Read the model definition and answer for the solid it produces. Units are mm, in the model's axes. A direction names the side the tool comes from. Coordinates: 2 decimals unless noted, no trailing zeros. Write each loop counter-clockwise with the first axis right and the second up, starting at its lowest first coordinate (ties: lowest second). Pieces come first, ordered by that corner, then holes. Notation, with made-up numbers: (71, 19.5) - (130, 19.5) arc R18 cw to (130, 41.5) - close; hole circle Ø1 at (-29.5, 47). An arc over 180 degrees is marked (long way). Return JSON: item names as keys, results as strings.
```python
from build123d import *

# Parameters (mm, degrees)
BOX458_W                    = 10
BOX458_H                    = 6
BOX458_DEPTH                = 2
BOX457_W                    = 10
BOX457_H                    = 6
BOX457_DEPTH                = 2
BOX459_W                    = 10
BOX459_H                    = 6
BOX459_DEPTH                = 2
BOX460_W                    = 10
BOX460_H                    = 6
BOX460_DEPTH                = 2
CYLINDER959_R               = 1.5
CYLINDER959_DEPTH           = 30
CYLINDER961_R               = 1.5
CYLINDER961_DEPTH           = 30
CYLINDER962_R               = 1.5
CYLINDER962_DEPTH           = 30
CYLINDER960_R               = 1.5
CYLINDER960_DEPTH           = 30
CYLINDER943_R               = 3
CYLINDER943_DEPTH           = 6
CYLINDER943_PLACEMENT_ANGLE = 45
CYLINDER945_R               = 3
CYLINDER945_DEPTH           = 6
CYLINDER947_R               = 3
CYLINDER947_DEPTH           = 6
CYLINDER947_PLACEMENT_ANGLE = 135
CYLINDER942_R               = 3
CYLINDER942_DEPTH           = 6
CYLINDER944_R               = 3
CYLINDER944_DEPTH           = 6
CYLINDER944_PLACEMENT_ANGLE = 225
CYLINDER946_R               = 3
CYLINDER946_DEPTH           = 6
CYLINDER941_R               = 3
CYLINDER941_DEPTH           = 6
CYLINDER941_PLACEMENT_ANGLE = 45
CYLINDER940_R               = 3
CYLINDER940_DEPTH           = 6
COMPOUND804_PLACEMENT_ANGLE = 22.5
CYLINDER934_R               = 1.5
CYLINDER934_DEPTH           = 40
CYLINDER934_PLACEMENT_ANGLE = 45
CYLINDER938_R               = 1.5
CYLINDER938_DEPTH           = 40
CYLINDER933_R               = 1.5
CYLINDER933_DEPTH           = 40
CYLINDER933_PLACEMENT_ANGLE = 135
CYLINDER935_R               = 1.5
CYLINDER935_DEPTH           = 40
CYLINDER939_R               = 1.5
CYLINDER939_DEPTH           = 40
CYLINDER939_PLACEMENT_ANGLE = 225
CYLINDER936_R               = 1.5
CYLINDER936_DEPTH           = 40
CYLINDER932_R               = 1.5
CYLINDER932_DEPTH           = 40
CYLINDER932_PLACEMENT_ANGLE = 45
CYLINDER937_R               = 1.5
CYLINDER937_DEPTH           = 40
COMPOUND803_PLACEMENT_ANGLE = 22.5
BOX435_W                    = 20
BOX435_H                    = 200
BOX435_DEPTH                = 20
BOX436_W                    = 20
BOX436_H                    = 200
BOX436_DEPTH                = 20
TUBE041_R                   = 54
TUBE041_R_2                 = 37
TUBE041_DEPTH               = 23


with BuildPart() as krychle458:
    # Box458 → Box458 (new body)
    with BuildSketch(Plane(origin=(55, 3, 54), x_dir=(-1, 0, 0), z_dir=(0, 0, 1))):
        with Locations((5, 3)):
            Rectangle(BOX458_W, BOX458_H)
    extrude(amount=BOX458_DEPTH)


with BuildPart() as krychle457:
    # Box457 → Box457 (new body)
    with BuildSketch(Plane(origin=(3, -55, 54), x_dir=(0, 1, 0), z_dir=(0, 0, 1))):
        with Locations((5, 3)):
            Rectangle(BOX457_W, BOX457_H)
    extrude(amount=BOX457_DEPTH)


with BuildPart() as krychle459:
    # Box459 → Box459 (new body)
    with BuildSketch(Plane(origin=(-55, -3, 54), x_dir=(1, 0, 0), z_dir=(0, 0, 1))):
        with Locations((5, 3)):
            Rectangle(BOX459_W, BOX459_H)
    extrude(amount=BOX459_DEPTH)


with BuildPart() as compound815:
    # Box460 → Box460 (new body)
    with BuildSketch(Plane(origin=(-3, 55, 54), x_dir=(0, -1, 0), z_dir=(0, 0, 1))):
        with Locations((5, 3)):
            Rectangle(BOX460_W, BOX460_H)
    extrude(amount=BOX460_DEPTH)

    # Compound815: union Krychle458, Krychle457, Krychle459
    add(krychle458.part)
    add(krychle457.part)
    add(krychle459.part)


with BuildPart() as obj1:
    # Cylinder959 → Cylinder959 (new body)
    with BuildSketch(Plane(origin=(50, 0, 35.5), x_dir=(-1, 0, 0), z_dir=(0, 0, 1))):
        Circle(CYLINDER959_R)
    extrude(amount=CYLINDER959_DEPTH)


with BuildPart() as obj2:
    # Cylinder961 → Cylinder961 (new body)
    with BuildSketch(Plane(origin=(0, -50, 35.5), x_dir=(0, 1, 0), z_dir=(0, 0, 1))):
        Circle(CYLINDER961_R)
    extrude(amount=CYLINDER961_DEPTH)


with BuildPart() as obj3:
    # Cylinder962 → Cylinder962 (new body)
    with BuildSketch(Plane(origin=(-50, 0, 35.5), x_dir=(1, 0, 0), z_dir=(0, 0, 1))):
        Circle(CYLINDER962_R)
    extrude(amount=CYLINDER962_DEPTH)


with BuildPart() as compound814:
    # Cylinder960 → Cylinder960 (new body)
    with BuildSketch(Plane(origin=(0, 50, 35.5), x_dir=(0, -1, 0), z_dir=(0, 0, 1))):
        Circle(CYLINDER960_R)
    extrude(amount=CYLINDER960_DEPTH)

    # Compound814: union obj1, obj2, obj3
    add(obj1.part)
    add(obj2.part)
    add(obj3.part)


with BuildPart() as obj4:
    # Cylinder943 → Cylinder943 (new body)
    with BuildSketch(Plane.XY):
        Circle(CYLINDER943_R)
    extrude(amount=CYLINDER943_DEPTH)


with BuildPart() as obj4_1:
    # Cylinder943 placement: moved
    add(obj4.part.moved(Location((29.698485, -29.698485, 33.5))).rotate(Axis((29.698485, -29.698485, 33.5), (0, 0, 1)), CYLINDER943_PLACEMENT_ANGLE))


with BuildPart() as obj5:
    # Cylinder945 → Cylinder945 (new body)
    with BuildSketch(Plane(origin=(42, 0, 33.5), x_dir=(0, 1, 0), z_dir=(0, 0, 1))):
        Circle(CYLINDER945_R)
    extrude(amount=CYLINDER945_DEPTH)


with BuildPart() as obj6:
    # Cylinder947 → Cylinder947 (new body)
    with BuildSketch(Plane.XY):
        Circle(CYLINDER947_R)
    extrude(amount=CYLINDER947_DEPTH)


with BuildPart() as obj6_1:
    # Cylinder947 placement: moved
    add(obj6.part.moved(Location((29.698485, 29.698485, 33.5))).rotate(Axis((29.698485, 29.698485, 33.5), (0, 0, 1)), CYLINDER947_PLACEMENT_ANGLE))


with BuildPart() as obj7:
    # Cylinder942 → Cylinder942 (new body)
    with BuildSketch(Plane(origin=(0, 42, 33.5), x_dir=(-1, 0, 0), z_dir=(0, 0, 1))):
        Circle(CYLINDER942_R)
    extrude(amount=CYLINDER942_DEPTH)


with BuildPart() as obj8:
    # Cylinder944 → Cylinder944 (new body)
    with BuildSketch(Plane.XY):
        Circle(CYLINDER944_R)
    extrude(amount=CYLINDER944_DEPTH)


with BuildPart() as obj8_1:
    # Cylinder944 placement: moved
    add(obj8.part.moved(Location((-29.698485, 29.698485, 33.5))).rotate(Axis((-29.698485, 29.698485, 33.5), (0, 0, 1)), CYLINDER944_PLACEMENT_ANGLE))


with BuildPart() as obj9:
    # Cylinder946 → Cylinder946 (new body)
    with BuildSketch(Plane(origin=(-42, 0, 33.5), x_dir=(0, -1, 0), z_dir=(0, 0, 1))):
        Circle(CYLINDER946_R)
    extrude(amount=CYLINDER946_DEPTH)


with BuildPart() as obj10:
    # Cylinder941 → Cylinder941 (new body)
    with BuildSketch(Plane.XY):
        Circle(CYLINDER941_R)
    extrude(amount=CYLINDER941_DEPTH)


with BuildPart() as obj10_1:
    # Cylinder941 placement: moved
    add(obj10.part.moved(Location((-29.698485, -29.698485, 33.5))).rotate(Axis((-29.698485, -29.698485, 33.5), (0, 0, -1)), CYLINDER941_PLACEMENT_ANGLE))


with BuildPart() as compound804:
    # Cylinder940 → Cylinder940 (new body)
    with BuildSketch(Plane(origin=(0, -42, 33.5), x_dir=(1, 0, 0), z_dir=(0, 0, 1))):
        Circle(CYLINDER940_R)
    extrude(amount=CYLINDER940_DEPTH)

    # Compound804: union obj4, obj5, obj6, obj7, obj8, obj9, obj10
    add(obj4_1.part)
    add(obj5.part)
    add(obj6_1.part)
    add(obj7.part)
    add(obj8_1.part)
    add(obj9.part)
    add(obj10_1.part)


with BuildPart() as compound804_1:
    # Compound804 placement: moved
    add(compound804.part.moved(Location((0, 0, 21))).rotate(Axis((0, 0, 21), (0, 0, 1)), COMPOUND804_PLACEMENT_ANGLE))


with BuildPart() as obj11:
    # Cylinder934 → Cylinder934 (new body)
    with BuildSketch(Plane.XY):
        Circle(CYLINDER934_R)
    extrude(amount=CYLINDER934_DEPTH)


with BuildPart() as obj11_1:
    # Cylinder934 placement: moved
    add(obj11.part.moved(Location((29.698485, -29.698485, 33.5))).rotate(Axis((29.698485, -29.698485, 33.5), (0, 0, 1)), CYLINDER934_PLACEMENT_ANGLE))


with BuildPart() as obj12:
    # Cylinder938 → Cylinder938 (new body)
    with BuildSketch(Plane(origin=(42, 0, 33.5), x_dir=(0, 1, 0), z_dir=(0, 0, 1))):
        Circle(CYLINDER938_R)
    extrude(amount=CYLINDER938_DEPTH)


with BuildPart() as obj13:
    # Cylinder933 → Cylinder933 (new body)
    with BuildSketch(Plane.XY):
        Circle(CYLINDER933_R)
    extrude(amount=CYLINDER933_DEPTH)


with BuildPart() as obj13_1:
    # Cylinder933 placement: moved
    add(obj13.part.moved(Location((29.698485, 29.698485, 33.5))).rotate(Axis((29.698485, 29.698485, 33.5), (0, 0, 1)), CYLINDER933_PLACEMENT_ANGLE))


with BuildPart() as obj14:
    # Cylinder935 → Cylinder935 (new body)
    with BuildSketch(Plane(origin=(0, 42, 33.5), x_dir=(-1, 0, 0), z_dir=(0, 0, 1))):
        Circle(CYLINDER935_R)
    extrude(amount=CYLINDER935_DEPTH)


with BuildPart() as obj15:
    # Cylinder939 → Cylinder939 (new body)
    with BuildSketch(Plane.XY):
        Circle(CYLINDER939_R)
    extrude(amount=CYLINDER939_DEPTH)


with BuildPart() as obj15_1:
    # Cylinder939 placement: moved
    add(obj15.part.moved(Location((-29.698485, 29.698485, 33.5))).rotate(Axis((-29.698485, 29.698485, 33.5), (0, 0, 1)), CYLINDER939_PLACEMENT_ANGLE))


with BuildPart() as obj16:
    # Cylinder936 → Cylinder936 (new body)
    with BuildSketch(Plane(origin=(-42, 0, 33.5), x_dir=(0, -1, 0), z_dir=(0, 0, 1))):
        Circle(CYLINDER936_R)
    extrude(amount=CYLINDER936_DEPTH)


with BuildPart() as obj17:
    # Cylinder932 → Cylinder932 (new body)
    with BuildSketch(Plane.XY):
        Circle(CYLINDER932_R)
    extrude(amount=CYLINDER932_DEPTH)


with BuildPart() as obj17_1:
    # Cylinder932 placement: moved
    add(obj17.part.moved(Location((-29.698485, -29.698485, 33.5))).rotate(Axis((-29.698485, -29.698485, 33.5), (0, 0, -1)), CYLINDER932_PLACEMENT_ANGLE))


with BuildPart() as compound803:
    # Cylinder937 → Cylinder937 (new body)
    with BuildSketch(Plane(origin=(0, -42, 33.5), x_dir=(1, 0, 0), z_dir=(0, 0, 1))):
        Circle(CYLINDER937_R)
    extrude(amount=CYLINDER937_DEPTH)

    # Compound803: union obj11, obj12, obj13, obj14, obj15, obj16, obj17
    add(obj11_1.part)
    add(obj12.part)
    add(obj13_1.part)
    add(obj14.part)
    add(obj15_1.part)
    add(obj16.part)
    add(obj17_1.part)


with BuildPart() as compound803_1:
    # Compound803 placement: moved
    add(compound803.part.rotate(Axis((0, 0, 0), (0, 0, 1)), COMPOUND803_PLACEMENT_ANGLE))


with BuildPart() as krychle435:
    # Box435 → Box435 (new body)
    with BuildSketch(Plane(origin=(-45, 28, 8), x_dir=(1, 0, 0), z_dir=(0, 0, 1))):
        with Locations((10, 100)):
            Rectangle(BOX435_W, BOX435_H)
    extrude(amount=BOX435_DEPTH)


with BuildPart() as compound795:
    # Box436 → Box436 (new body)
    with BuildSketch(Plane(origin=(25, 28, 8), x_dir=(1, 0, 0), z_dir=(0, 0, 1))):
        with Locations((10, 100)):
            Rectangle(BOX436_W, BOX436_H)
    extrude(amount=BOX436_DEPTH)

    # Compound795: union Krychle435
    add(krychle435.part)


with BuildPart() as compound795_1:
    # Compound795 placement: moved
    add(compound795.part.moved(Location((0, 2, 32))))


with BuildPart() as cut407:
    # Tube041 → Tube041 (new body)
    with BuildSketch(Plane.XY.offset(37)):
        Circle(TUBE041_R)
        Circle(TUBE041_R_2, mode=Mode.SUBTRACT)
    extrude(amount=TUBE041_DEPTH)

    # Cut393: cut Compound795
    add(compound795_1.part, mode=Mode.SUBTRACT)

    # Cut395: cut Compound803
    add(compound803_1.part, mode=Mode.SUBTRACT)

    # Cut396: cut Compound804
    add(compound804_1.part, mode=Mode.SUBTRACT)

    # Cut406: cut Compound814
    add(compound814.part, mode=Mode.SUBTRACT)

    # Cut407: cut Compound815
    add(compound815.part, mode=Mode.SUBTRACT)


solid = cut407.part
```
(1) Flat-ended cylindrical pins translate along their axes: P1, Ø5, axis at x = -38, y = -16.5, coming from the +Z side; P2, Ø2, axis at x = 32, z = 57, coming from the +Y side; P3, Ø0.6, axis at y = -0.5, z = 55.5, coming from the +X side; P4, Ø1.5, axis at y = 3.5, z = 41.5, coming from the -X side. Find the tip coordinate at first contact, or state that the pin passes through.
Answer:
{"P1": "z = 60", "P2": "y = 30", "P3": "x = 45", "P4": "x = -53.93"}
(2) Determine the mould class of faces 6 (the face through (35, 30, 50)), 7 (the face through (-37, -16, 54.5)), 8 (the face through (-1.4, -48.6, 54)) for opening direction Y: +Y half, -Y half, draft (parallel to the pull), parting line (faces both ways), or undercut.
Answer:
{"face 6": "+Y half", "face 7": "undercut", "face 8": "draft"}
(3) Straight lines are drawn through the part: line 1 (Y direction, x = 40, z = 44); line 2 (Y direction, x = -17, z = 46.5); line 3 (Y direction, x = -39, z = 57). For each, find the intervals that lie inside material, in ascending order. Write a range as from..to.
Answer:
{"line 1": "-36.28..-16.98, -15.17..15.17, 16.98..30", "line 2": "-51.25..-39.98, -37.62..-32.86, 32.86..37.62, 39.98..51.25", "line 3": "-37.35..-19.07, -13.08..13.08, 19.07..30"}
(4) Which of the six approach directions +Z, -Z, +X, -X, +Y, -Y give full straight-line access (tool end or side, diameter ignored) to faces 1 (the face through (-48.6, 1.4, 54)), 2 (the face through (18.372, -36.875, 57.212)), 3 (the face through (-1.4, -48.6, 56)), 4 (the face through (25, 39, 50)), 5 (the face through (-25, 39, 50))?
Answer:
{"face 1": "-X", "face 2": "+Z", "face 3": "-Y", "face 4": "+Z, +X, +Y", "face 5": "+Z, -X, +Y"}
(5) A cutting plane is placed at C-C (y = -50). Determine the outline of the cut face in (x, z), and give its area (3 significant figures).
Answer:
{"outline": "(-20.4, 37) - (-1.5, 37) - (-1.5, 54) - (-3, 54) - (-3, 56) - (-1.5, 56) - (-1.5, 60) - (-20.4, 60) - close; (1.5, 37) - (20.4, 37) - (20.4, 60) - (1.5, 60) - (1.5, 56) - (3, 56) - (3, 54) - (1.5, 54) - close", "area": "863 mm²"}
(6) A cutting plane is placed at A-A (x = 0). State how many separate pieces and enclosed holes the cut face has, and give its area (3 significant figures).
Answer:
{"separate pieces": "6", "enclosed holes": "0", "area": "620 mm²"}
